```python
from build123d import *

# Parameters (mm, degrees)
SKETCH1_W           = 33.5
SKETCH1_H           = 30
BOSS_EXTRUDE1_DEPTH = 4.53
BOSS_EXTRUDE2_DEPTH = 5
FILLET1_R           = 2
FILLET3_R           = 0.8


with BuildPart() as part:
    # Sketch1 → Boss-Extrude1 (new body)
    with BuildSketch(Plane(origin=(0, 0, 0), x_dir=(1, 0, 0), z_dir=(0, 1, 0))):
        Rectangle(SKETCH1_W, SKETCH1_H)
    extrude(amount=BOSS_EXTRUDE1_DEPTH)

    # Sketch2 → Boss-Extrude2 (add)
    with BuildSketch(Plane(origin=(0, 4.53, 0), x_dir=(1, 0, 0), z_dir=(0, 1, 0))):
        Polygon((-14.75, 5), (-16.75, 5), (-16.75, -5), (-14.75, -5), (-14.75, -1), (14.75, -1), (14.75, -5), (16.75, -5), (16.75, 5), (14.75, 5), (14.75, 1), (-14.75, 1), align=None)
    extrude(amount=BOSS_EXTRUDE2_DEPTH)

    # Fillet1
    fillet1_edges = [part.edges().sort_by_distance(p)[0] for p in [
        (16.75, 2.265, 15),
        (-16.75, 2.265, 15),
        (-16.75, 2.265, -15),
        (16.75, 2.265, -15),
    ]]
    fillet(fillet1_edges, radius=FILLET1_R)

    # Fillet3
    fillet3_edges = [part.edges().sort_by_distance(p)[0] for p in [
        (14.75, 4.53, 3),
        (14.75, 7.03, 1),
        (15.75, 4.53, 5),
        (14.75, 7.03, 5),
        (15.75, 9.53, -5),
        (14.75, 9.53, -3),
        (14.75, 7.03, -5),
        (0, 9.53, -1),
        (14.75, 7.03, -1),
        (-14.75, 9.53, -3),
        (-14.75, 7.03, -1),
        (-15.75, 9.53, -5),
        (-14.75, 7.03, -5),
        (-15.75, 4.53, 5),
        (-14.75, 4.53, 3),
        (-14.75, 7.03, 5),
        (0, 4.53, 1),
        (-14.75, 7.03, 1),
        (14.75, 9.53, 3),
        (15.75, 9.53, 5),
        (-15.75, 9.53, 5),
        (-14.75, 9.53, 3),
        (0, 9.53, 1),
        (-15.75, 4.53, -5),
        (-14.75, 4.53, -3),
        (0, 4.53, -1),
        (14.75, 4.53, -3),
        (15.75, 4.53, -5),
    ]]
    fillet(fillet3_edges, radius=FILLET3_R)


solid = part.part
```
Can you work these out from the model? Positions are in its coordinate system, mm. A direction names the side the tool comes from. Round coordinates to 2 decimals unless told otherwise and drop trailing zeros. Order: outer loops, then holes, each group sorted by start corner. A loop starts at its lowest first (then second) coordinate and runs counter-clockwise, first axis right, second up. Notation, with made-up numbers: (-8.75, 60.25) -> (7.25, 60.25) arc R29 cw to (7.25, 99.25) -> close; hole circle Ø8 at (15, 57). An arc over 180 degrees is marked (long way). Return JSON: item names as keys, results as strings. Group by question number.
1. We'd pull the mould along X, two halves only. Please class faces 1 (the face through (16.15, 2.3, 14.43)), 2 (the face through (14.51, 7.05, 1.23)), 3 (the face through (0, 0, 0)): released by +X, released by -X, zero draft, split by the parting line, or undercut.
2. Which directions (+Z, -Z, +X, -X, +Y, -Y) give clear straight access to the entire face, cutting with the end or side of a thin tool? Please do faces 4 (the face through (16, 7, -5)), 5 (the face through (-14.75, 7, 3)), 6 (the face through (-14.99, 7.05, -4.77)).
3. If we section it at C-C, the plane z = 11.5: Write out the boundary of the cut face in (x, y), then the cut area to 3 significant figures.
4. Will these pins go through, and if not, where does the flat tip stop? pin 1 (0.6 mm diameter, centred on x = 16, y = 7, fed in from -Z); pin 2 (2.5 mm diameter, centred on x = -6.5, y = 7, fed in from -Z); pin 3 (8 mm diameter, centred on x = -6, z = 4, fed in from +Y); pin 4 (3.5 mm diameter, centred on x = 0, y = 8, fed in from +Z).
5. If we section it at B-B, the plane y = 6.25: Write out the boundary of the cut face in (x, z).
6. I need wall thicknesses on line 1 (Z direction, x = 14, y = 7.5); line 2 (Y direction, x = 9, z = -6); line 3 (X direction, y = 9, z = 4). Which ranges of each line are inside material? Lowest first, please. Write a range as [from, to].
7. If we section it at A-A, the plane x = -13: Write out the boundary of the cut face in (y, z).
Output values:
{
 "1": {"face 1": "released by +X", "face 2": "undercut", "face 3": "zero draft"},
 "2": {"face 4": "-Z, +X, -X, +Y", "face 5": "+Z, +Y", "face 6": "-Z, +Y"},
 "3": {"outline": "(-16.75, 0) -> (16.75, 0) -> (16.75, 4.53) -> (-16.75, 4.53) -> close", "area": "152 mm²"},
 "4": {"pin 1": "z = -5", "pin 2": "z = -1", "pin 3": "y = 9.53", "pin 4": "z = 1"},
 "5": {"outline": "(-16.75, -5) -> (-15.55, -5) arc R0.8 ccw to (-14.75, -4.2) -> (-14.75, -1.8) arc R0.8 cw to (-13.95, -1) -> (13.95, -1) arc R0.8 cw to (14.75, -1.8) -> (14.75, -4.2) arc R0.8 ccw to (15.55, -5) -> (16.75, -5) -> (16.75, 5) -> (15.55, 5) arc R0.8 ccw to (14.75, 4.2) -> (14.75, 1.8) arc R0.8 cw to (13.95, 1) -> (-13.95, 1) arc R0.8 cw to (-14.75, 1.8) -> (-14.75, 4.2) arc R0.8 ccw to (-15.55, 5) -> (-16.75, 5) -> close"},
 "6": {"line 1": "[-1, 1]", "line 2": "[0, 4.53]", "line 3": "[-16.75, -14.8], [14.8, 16.75]"},
 "7": {"outline": "(0, -15) -> (4.53, -15) -> (4.53, -1.8) arc R0.8 cw to (5.33, -1) -> (8.73, -1) arc R0.8 ccw to (9.53, -0.2) -> (9.53, 0.2) arc R0.8 ccw to (8.73, 1) -> (5.33, 1) arc R0.8 cw to (4.53, 1.8) -> (4.53, 15) -> (0, 15) -> close"}
}
